```python
from build123d import *

# Parameters (mm, degrees)
SKETCH1_W          = 30
SKETCH1_H          = 15
BASE_FLANGE1_DEPTH = 0.67
EDGE_FLANGE1_DEPTH = 30
SKETCH7_R          = 1.7
CUT_EXTRUDE1_DEPTH = 10
FILLET1_R          = 2


# Sheet-metal steps are written as plain solids
with BuildPart() as part:
    # Sketch1 → Base-Flange1 (new body)
    with BuildSketch(Plane(origin=(0, 0, 0), x_dir=(1, 0, 0), z_dir=(0, 1, 0))):
        with Locations((15, -7.5)):
            Rectangle(SKETCH1_W, SKETCH1_H)
    extrude(amount=-BASE_FLANGE1_DEPTH)

    # Edge-Flange1 section (across the edge) → Edge-Flange1 (add)
    with BuildSketch(Plane(origin=(0, 0, 15.7366), x_dir=(0, 0, -1), z_dir=(1, 0, 0))):
        with BuildLine():
            Line((-0.67, 0.7366), (-0.67, 20))
            Line((-0.67, 20), (0, 20))
            Line((0, 20), (0, 0.7366))
            ThreePointArc((0, 0.7366), (0.215745145, 0.215745145), (0.7366, 0))
            Line((0.7366, 0), (0.7366, -0.67))
            ThreePointArc((0.7366, -0.67), (-0.258016398, -0.258016398), (-0.67, 0.7366))
        make_face()
    extrude(amount=EDGE_FLANGE1_DEPTH)

    # Sketch7 → Cut-Extrude1 (cut)
    with BuildSketch(Plane(origin=(0, 0, 0), x_dir=(1, 0, 0), z_dir=(0, 1, 0))):
        with Locations(Location((15, -7.9066, 0), (0, 0, 270))):
            Circle(SKETCH7_R)
    extrude(amount=-CUT_EXTRUDE1_DEPTH, mode=Mode.SUBTRACT)

    # Fillet1
    fillet1_edges = [part.edges().sort_by_distance(p)[0] for p in [
        (0, 20, 16.0716),
        (30, 20, 16.0716),
        (0, -0.335, 0),
        (30, -0.335, 0),
    ]]
    fillet(fillet1_edges, radius=FILLET1_R)


solid = part.part
```
Input: part model. Units: mm. Frame: model coordinates. A direction names the side the tool comes from. Give positions to 0.01 mm unless a question says otherwise; leave off trailing zeros. Order: outer loops, then holes, each group sorted by start corner. A loop starts at its lowest first (then second) coordinate and runs counter-clockwise, first axis right, second up. Notation, with made-up numbers: (78, -10) - (134, -10) arc R16 ccw to (134, 9) - close; hole circle Ø10 at (-11, 53.5). An arc over 180 degrees is marked (long way). Use a Markdown table: item, result.
(1) Pin query (flat end, axial travel): pin 1 (6 mm diameter, centred on x = 19, y = 12, fed in from -Z); pin 2 (4.5 mm diameter, centred on x = 10.5, z = 5.5, fed in from +Y). Return the tip coordinate at first contact, or that it passes through.
Computed values:
| item | result |
|---|---|
| pin 1 | stops at z = 15.74 |
| pin 2 | stops at y = 0 |
(2) Section query D-D (z = 12.5). Output: boundary loops of the cut face in (x, y), then the cut area to 3 significant figures.
Computed values:
| item | result |
|---|---|
| outline | (0, -0.67) - (30, -0.67) - (30, 0) - (0, 0) - close |
| area | 20.1 mm2 |
(3) Section query A-A (x = 15). Output: boundary loops of the cut face in (y, z), then the cut area to 3 significant figures.
Computed values:
| item | result |
|---|---|
| outline | (-0.67, 0) - (0, 0) - (0, 6.21) - (-0.67, 6.21) - close; (-0.67, 9.61) - (0, 9.61) - (0, 15) arc R0.74 cw to (0.74, 15.74) - (20, 15.74) - (20, 16.41) - (0.74, 16.41) arc R1.41 ccw to (-0.67, 15) - close |
| area | 21.8 mm2 |
(4) Line query: line 1 (Z direction, x = 17.5, y = 16); line 2 (Y direction, x = 28.75, z = 11.25); line 3 (Y direction, x = 24, z = 15.25). Output: solid intervals per line, ascending. Write a range as from..to.
Computed values:
| item | result |
|---|---|
| line 1 | z = 15.74..16.41 |
| line 2 | y = -0.67..0 |
| line 3 | y = -0.65..0.04 |
(5) Section query C-C (x = 25.5). Output: boundary loops of the cut face in (y, z).
Computed values:
| item | result |
|---|---|
| outline | (-0.67, 0) - (0, 0) - (0, 15) arc R0.74 cw to (0.74, 15.74) - (20, 15.74) - (20, 16.41) - (0.74, 16.41) arc R1.41 ccw to (-0.67, 15) - close |
(6) Access query for faces 4 (the flat face through (15, 0, 6)), 5 (the cylindrical face through (29.4, 19.43, 16.07)). Directions: +Z, -Z, +X, -X, +Y, -Y. A direction counts if a zero-diameter tool reaches every point of the face in a straight line with its end or side. Return the directions, or none.
Computed values:
| item | result |
|---|---|
| face 4 | -Z, +X, -X, +Y |
| face 5 | +Z, -Z, +X, +Y |
(7) Section query B-B (z = 9). Output: boundary loops of the cut face in (x, y), then the cut area to 3 significant figures.
Computed values:
| item | result |
|---|---|
| outline | (0, -0.67) - (13.7, -0.67) - (13.7, 0) - (0, 0) - close; (16.3, -0.67) - (30, -0.67) - (30, 0) - (16.3, 0) - close |
| area | 18.4 mm2 |
(8) Draft query along Z for faces 1 (the cylindrical face through (14.349, -0.33, 9.477)), 2 (the flat face through (15, -0.67, 6)), 3 (the flat face through (15, 11, 15.737)). Return one class per face: released by +Z, released by -Z, zero draft, split by the parting line, or undercut.
Computed values:
| item | result |
|---|---|
| face 1 | undercut |
| face 2 | zero draft |
| face 3 | released by -Z |
